Design review of the part built by this model. Coordinates are the model's own, in mm. Face numbers are marked on the shaded views. Coordinates: 2 decimals unless noted, no trailing zeros. Write each loop counter-clockwise with the first axis right and the second up, starting at its lowest first coordinate (ties: lowest second). Pieces come first, ordered by that corner, then holes.
Q1. Mouldability with a two-part tool opening along X and no side actions: class the marked faces 1, 2 and 3 as pulls with the +X half, pulls with the -X half, needs draft (parallel to the pull), parting line crosses it, or undercut.
Q2. Take a section at C-C (y = 7.5). Give the boundary of the cut face in (x, z).
Q3. Insertion check: pin 1 (3.5 mm diameter, centred on x = 40, y = 17, fed in from -Z); pin 2 (10 mm diameter, centred on y = 32.5, z = -3.5, fed in from -X); pin 3 (6 mm diameter, centred on y = 59, z = -5, fed in from -X); pin 4 (2 mm diameter, centred on x = 10.5, y = -18.19, fed in from -Z). Each pin has a flat end and moves straight along its axis. Give the tip position at first contact, or say it passes through.
Q4. Take a section at D-D (z = -18). Give the boundary of the cut face in (x, y).
Q5. For probe 1 along Y at (x, z) = (40, -29); probe 2 along X at (y, z) = (-17, -30); probe 3 along X at (y, z) = (-4, -15.5), list the stretches that pass through material, from the lowest coordinate up.
Q6. Take a section at B-B (x = 53.5). Give the boundary of the cut face in (y, z).
Q7. Take a section at A-A (z = -26.5). Give the boundary of the cut face in (x, y).
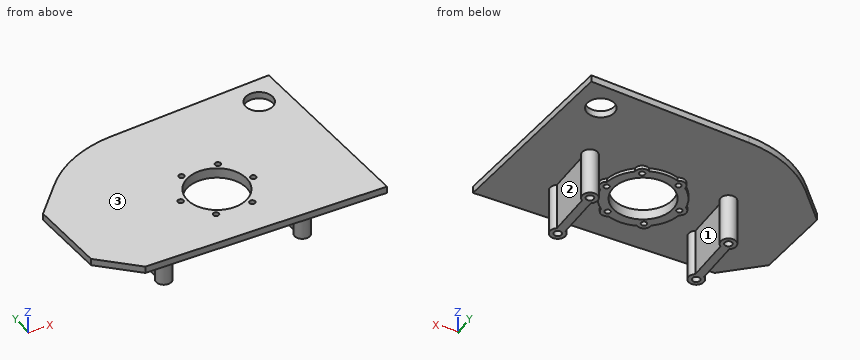
```python
from build123d import *

# Parameters (mm, degrees)
SKETCH2_R           = 8
SKETCH2_R_2         = 17.5
BOSS_EXTRUDE2_DEPTH = 4
SKETCH2_3_R         = 17.5
BOSS_EXTRUDE3_DEPTH = 6
SKETCH2_6_R         = 1.65
CUT_EXTRUDE1_DEPTH  = 113.610704204
BOSS_EXTRUDE4_DEPTH = 31.5
CUT_EXTRUDE2_START  = -31.5
SKETCH2_8_R         = 2.2
CUT_EXTRUDE2_DEPTH  = 7


with BuildPart() as part:
    # Sketch2 → Boss-Extrude2 (new body)
    with BuildSketch(Plane.XY):
        with BuildLine():
            Line((-87.139041318, 24.298867192), (-84, -20.59151507))
            Line((-84, -20.59151507), (-63, -39.5))
            Line((-63, -39.5), (76.577227286, -39.5))
            Line((76.577227286, -39.5), (68.844921224, 71.077128384))
            Line((68.844921224, 71.077128384), (-26, 64.444925414))
            ThreePointArc((-26, 64.444925414), (-50.392441883, 57.90899031), (-70.560315786, 42.711407248))
            Line((-70.560315786, 42.711407248), (-87.139041318, 24.298867192))
        make_face()
        with Locations((54, 54)):
            Circle(SKETCH2_R, mode=Mode.SUBTRACT)
        Circle(SKETCH2_R_2, mode=Mode.SUBTRACT)
    extrude(amount=-BOSS_EXTRUDE2_DEPTH)

    # Sketch2<3> → Boss-Extrude3 (add)
    with BuildSketch(Plane.XY):
        with BuildLine():
            ThreePointArc((-14.486986043, 17.864132652), (-19.918584287, 11.5), (-22.714285714, 3.614031612))
            ThreePointArc((-22.714285714, 3.614031612), (-25, 0), (-22.714285714, -3.614031612))
            ThreePointArc((-22.714285714, -3.614031612), (-19.918584287, -11.5), (-14.486986043, -17.864132652))
            ThreePointArc((-14.486986043, -17.864132652), (-12.5, -21.650635095), (-8.227299671, -21.478164263))
            ThreePointArc((-8.227299671, -21.478164263), (0, -23), (8.227299671, -21.478164263))
            ThreePointArc((8.227299671, -21.478164263), (12.5, -21.650635095), (14.486986043, -17.864132652))
            ThreePointArc((14.486986043, -17.864132652), (19.918584287, -11.5), (22.714285714, -3.614031612))
            ThreePointArc((22.714285714, -3.614031612), (25, 0), (22.714285714, 3.614031612))
            ThreePointArc((22.714285714, 3.614031612), (19.918584287, 11.5), (14.486986043, 17.864132652))
            ThreePointArc((14.486986043, 17.864132652), (12.5, 21.650635095), (8.227299671, 21.478164263))
            ThreePointArc((8.227299671, 21.478164263), (0, 23), (-8.227299671, 21.478164263))
            ThreePointArc((-8.227299671, 21.478164263), (-12.5, 21.650635095), (-14.486986043, 17.864132652))
        make_face()
        Circle(SKETCH2_3_R, mode=Mode.SUBTRACT)
    extrude(amount=-BOSS_EXTRUDE3_DEPTH)

    # Sketch2<6> → Cut-Extrude1 (cut, through all)
    with BuildSketch(Plane.XY):
        with Locations((-10.5, 18.186533479)):
            Circle(SKETCH2_6_R)
        with Locations((10.5, 18.186533479)):
            Circle(SKETCH2_6_R)
        with Locations((21, 0)):
            Circle(SKETCH2_6_R)
        with Locations((10.5, -18.186533479)):
            Circle(SKETCH2_6_R)
        with Locations((-10.5, -18.186533479)):
            Circle(SKETCH2_6_R)
        with Locations((-21, 0)):
            Circle(SKETCH2_6_R)
    extrude(amount=-CUT_EXTRUDE1_DEPTH, mode=Mode.SUBTRACT)

    # Sketch2<7> → Boss-Extrude4 (add)
    with BuildSketch(Plane.XY):
        with BuildLine():
            Line((-42.5, 13.258342613), (-42.5, -13.258342613))
            ThreePointArc((-42.5, -13.258342613), (-40, -21.5), (-37.5, -13.258342613))
            Line((-37.5, -13.258342613), (-37.5, 13.258342613))
            ThreePointArc((-37.5, 13.258342613), (-40, 21.5), (-42.5, 13.258342613))
        make_face()
        with BuildLine():
            Line((42.5, 13.258342613), (42.5, -13.258342613))
            ThreePointArc((42.5, -13.258342613), (40, -21.5), (37.5, -13.258342613))
            Line((37.5, -13.258342613), (37.5, 13.258342613))
            ThreePointArc((37.5, 13.258342613), (40, 21.5), (42.5, 13.258342613))
        make_face()
    extrude(amount=-BOSS_EXTRUDE4_DEPTH)

    # Sketch2<8> → Cut-Extrude2 (cut)
    with BuildSketch(Plane.XY.offset(CUT_EXTRUDE2_START)):
        with Locations(Location((-40, 17, 0), (0, 0, 180))):
            Circle(SKETCH2_8_R)
        with Locations(Location((-40, -17, 0), (0, 0, 180))):
            Circle(SKETCH2_8_R)
        with Locations(Location((40, 17, 0), (0, 0, 180))):
            Circle(SKETCH2_8_R)
        with Locations(Location((40, -17, 0), (0, 0, 180))):
            Circle(SKETCH2_8_R)
    extrude(amount=CUT_EXTRUDE2_DEPTH, mode=Mode.SUBTRACT)


solid = part.part
```
Response:
1. face 1: undercut
1. face 2: pulls with the +X half
1. face 3: needs draft
2. outline: (-85.96, -4) - (-42.5, -4) - (-42.5, -31.5) - (-37.5, -31.5) - (-37.5, -4) - (-21.74, -4) - (-21.74, -6) - (-15.81, -6) - (-15.81, 0) - (-85.96, 0) - close; (15.81, -6) - (21.74, -6) - (21.74, -4) - (37.5, -4) - (37.5, -31.5) - (42.5, -31.5) - (42.5, -4) - (73.29, -4) - (73.29, 0) - (15.81, 0) - close
3. pin 1: stops at z = -24.5
3. pin 2: stops at x = -84.26
3. pin 3: stops at x = -53.71
3. pin 4: passes through
4. outline: (-42.5, -13.26) arc R4.5 ccw (long way) to (-37.5, -13.26) - (-37.5, 13.26) arc R4.5 ccw (long way) to (-42.5, 13.26) - close; (37.5, -13.26) arc R4.5 ccw (long way) to (42.5, -13.26) - (42.5, 13.26) arc R4.5 ccw (long way) to (37.5, 13.26) - close
5. probe 1: y = -21.5 to -19.2, -14.8 to 14.8, 19.2 to 21.5
5. probe 2: x = -44.5 to -42.2, -37.8 to -35.5, 35.5 to 37.8, 42.2 to 44.5
5. probe 3: x = -42.5 to -37.5, 37.5 to 42.5
6. outline: (-39.5, -4) - (46.02, -4) - (46.02, 0) - (-39.5, 0) - close; (61.98, -4) - (70, -4) - (70, 0) - (61.98, 0) - close
7. outline: (-42.5, -13.26) arc R4.5 ccw (long way) to (-37.5, -13.26) - (-37.5, 13.26) arc R4.5 ccw (long way) to (-42.5, 13.26) - close; (37.5, -13.26) arc R4.5 ccw (long way) to (42.5, -13.26) - (42.5, 13.26) arc R4.5 ccw (long way) to (37.5, 13.26) - close; hole circle Ø4.4 at (-40, -17); hole circle Ø4.4 at (-40, 17); hole circle Ø4.4 at (40, -17); hole circle Ø4.4 at (40, 17)
